Check sheet for the drawn part. Datum: minimum x, y, z corner. Units: mm. Give positions to 0.01 mm unless a question says otherwise; leave off trailing zeros. Write each loop counter-clockwise with the first axis right and the second up, starting at its lowest first coordinate (ties: lowest second). Pieces come first, ordered by that corner, then holes. Notation, with made-up numbers: (51, -18.5) - (83, -18.5) arc R15 ccw to (83, -5.5) - close; hole circle Ø3 at (74.5, -3.5). An arc over 180 degrees is marked (long way). Answer as a JSON object with one key per item and string values. Group by question number.
Item 1: Go/stop test with flat-tipped pins: pin 1 (2.5 mm diameter, centred on x = 2.7, y = 2.5, fed in from +Z); pin 2 (1.3 mm diameter, centred on x = 10.7, y = 2.5, fed in from -Z). Record where each tip stops, or that it passes through.
Item 2: Sectioned sample at B-B, the plane y = 2.5. Record the boundary of the cut face in (x, z).
Item 3: Scan lines: line 1 along Y through (x, z) = (10.7, 2.65); line 2 along Y through (x, z) = (6.75, 3.2); line 3 along X through (y, z) = (2.75, 2.4). Record each from-to range of solid material in increasing order. Write a range as [from, to].
Item 4: Sectioned sample at A-A, the plane x = 10.7. Record the boundary of the cut face in (y, z), and give its area (3 significant figures).
Item 5: Draft check along X on the marked faces 1, 2, 3 and 4. Enter one of: +X half, -X half, draft (parallel to the pull), parting line (faces both ways), or undercut.
Item 6: Sectioned sample at D-D, the plane x = 6.7. Record the boundary of the cut face in (y, z).
Item 7: Sectioned sample at C-C, the plane z = 3.6. Record the boundary of the cut face in (x, y), and give its area (3 significant figures).
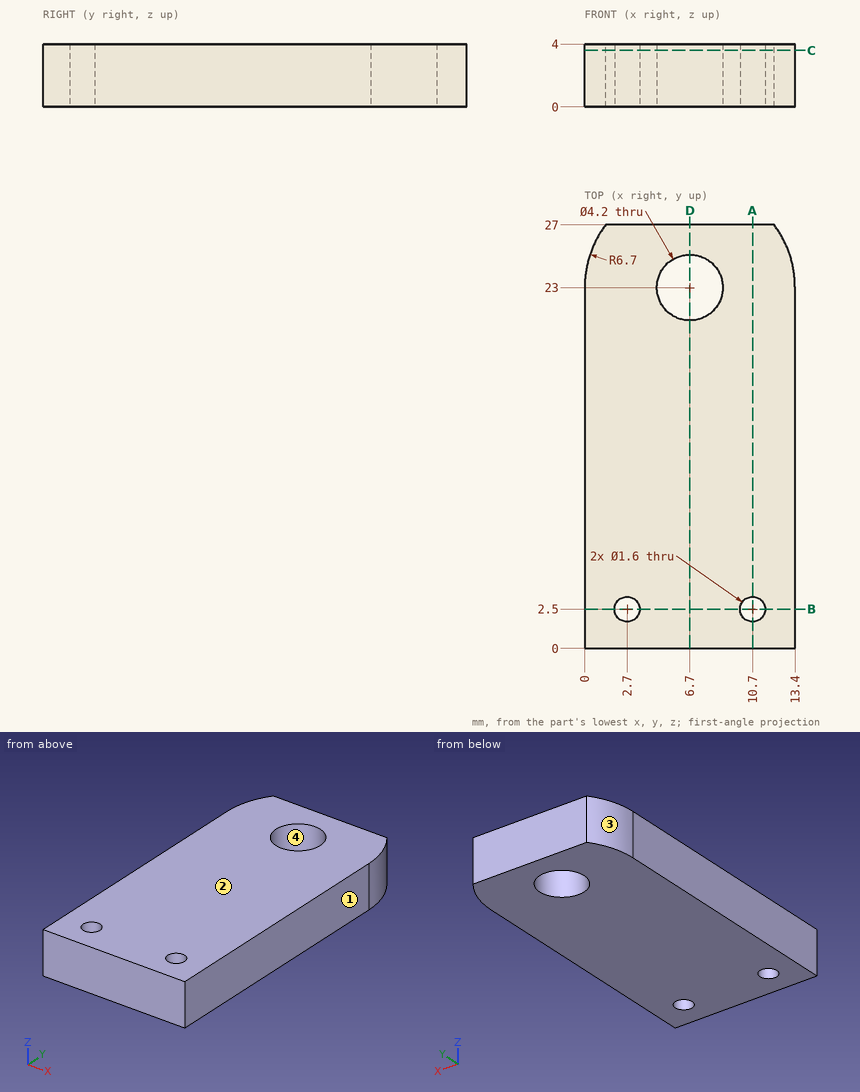
Geometry check:
{
 "1": {"pin 1": "z = 4", "pin 2": "through"},
 "2": {"outline": "(0, 0) - (1.9, 0) - (1.9, 4) - (0, 4) - close; (3.5, 0) - (9.9, 0) - (9.9, 4) - (3.5, 4) - close; (11.5, 0) - (13.4, 0) - (13.4, 4) - (11.5, 4) - close"},
 "3": {"line 1": "[0, 1.7], [3.3, 27]", "line 2": "[0, 20.9], [25.1, 27]", "line 3": "[0, 1.94], [3.46, 9.94], [11.46, 13.4]"},
 "4": {"outline": "(0, 0) - (1.7, 0) - (1.7, 4) - (0, 4) - close; (3.3, 0) - (27, 0) - (27, 4) - (3.3, 4) - close", "area": "102 mm^2"},
 "5": {"face 1": "+X half", "face 2": "draft", "face 3": "-X half", "face 4": "undercut"},
 "6": {"outline": "(0, 0) - (20.9, 0) - (20.9, 4) - (0, 4) - close; (25.1, 0) - (27, 0) - (27, 4) - (25.1, 4) - close"},
 "7": {"outline": "(0, 0) - (13.4, 0) - (13.4, 23) arc R6.7 ccw to (12.07, 27) - (1.33, 27) arc R6.7 ccw to (0, 23) - close; hole circle Ø1.6 at (2.7, 2.5); hole circle Ø4.2 at (6.7, 23); hole circle Ø1.6 at (10.7, 2.5)", "area": "341 mm^2"}
}
